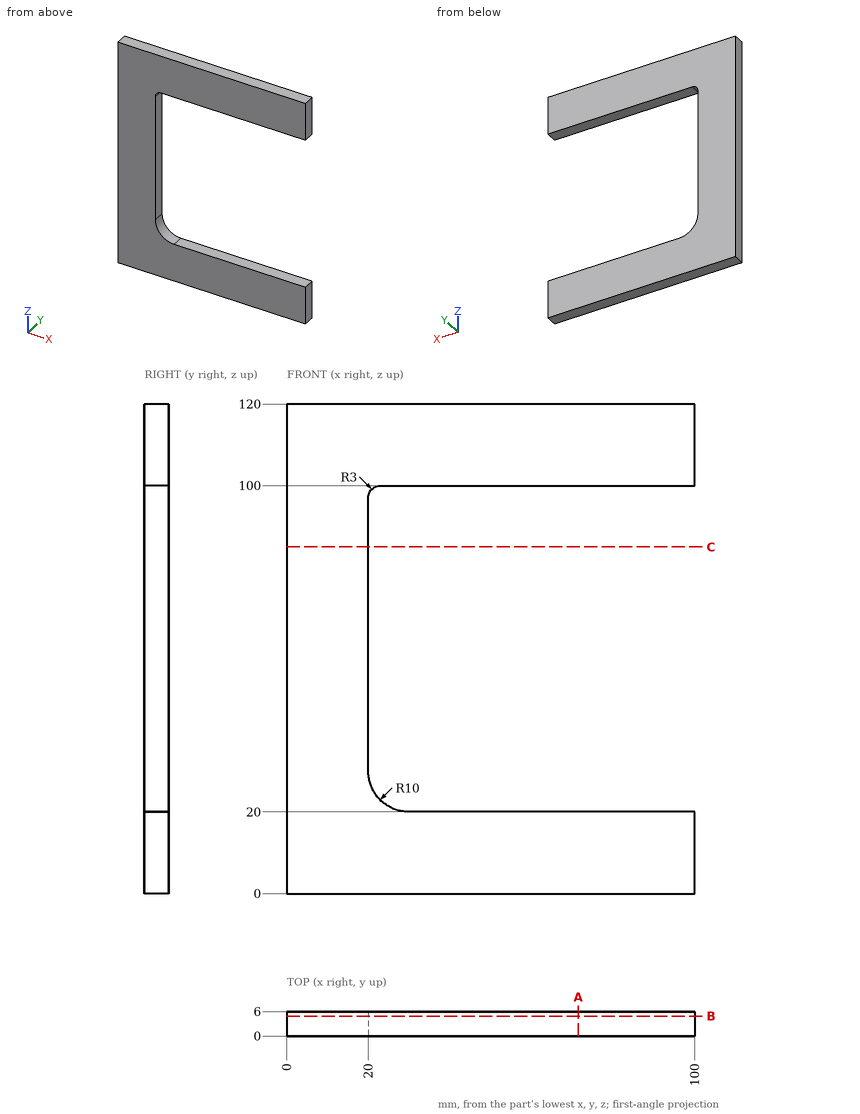
Here's the drawing with two shaded views (mm, measured from the low corner). I have some questions. Round coordinates to 2 decimals unless told otherwise and drop trailing zeros. Loops run counter-clockwise (first coordinate to the right, second up) from the corner with the lowest first, then second, coordinate; pieces in that order, holes last.
Item 1: Please list where these lines run through material, in increasing order: L1, parallel to Z at x = 88, y = 5.2; L2, parallel to X at y = 4.2, z = 40.5; L3, parallel to Z at x = 26, y = 2.75.
Item 2: Suppose I cut it at C-C, the plane z = 85. Write out the boundary of the cut face in (x, y), then the cut area to 3 significant figures.
Item 3: Suppose I cut it at A-A, the plane x = 71.5. Write out the boundary of the cut face in (y, z), then the cut area to 3 significant figures.
Item 4: Will this pin go through, and if not, where does the flat tip stop? pin 1 Ø1 at (y, z) = (1.5, 23) entering from +X.
Item 5: Suppose I cut it at B-B, the plane y = 4.9. Write out the boundary of the cut face in (x, z), then the cut area to 3 significant figures.
Reported:
1. L1: z = 0 to 20, 100 to 120
1. L2: x = 0 to 20
1. L3: z = 0 to 20.83, 100 to 120
2. outline: (0, 0) - (20, 0) - (20, 6) - (0, 6) - close
2. area: 120 mm2
3. outline: (0, 0) - (6, 0) - (6, 20) - (0, 20) - close; (0, 100) - (6, 100) - (6, 120) - (0, 120) - close
3. area: 240 mm2
4. pin 1: stops at x = 23.39
5. outline: (0, 0) - (100, 0) - (100, 20) - (30, 20) arc R10 cw to (20, 30) - (20, 97) arc R3 cw to (23, 100) - (100, 100) - (100, 120) - (0, 120) - close
5. area: 5,620 mm2
